Can you work these out from the drawing? Everything is in mm from the part's minimum corner. Coordinates: 2 decimals unless noted, no trailing zeros. Order: outer loops, then holes, each group sorted by start corner. A loop starts at its lowest first (then second) coordinate and runs counter-clockwise, first axis right, second up. Notation, with made-up numbers: M 39.5,65 L 80.5,65 A22 ccw 80.5,97 Z; hole C 85,65 d9. An arc over 180 degrees is marked long. Answer as CSV lines item,"result". Start each with the question number.
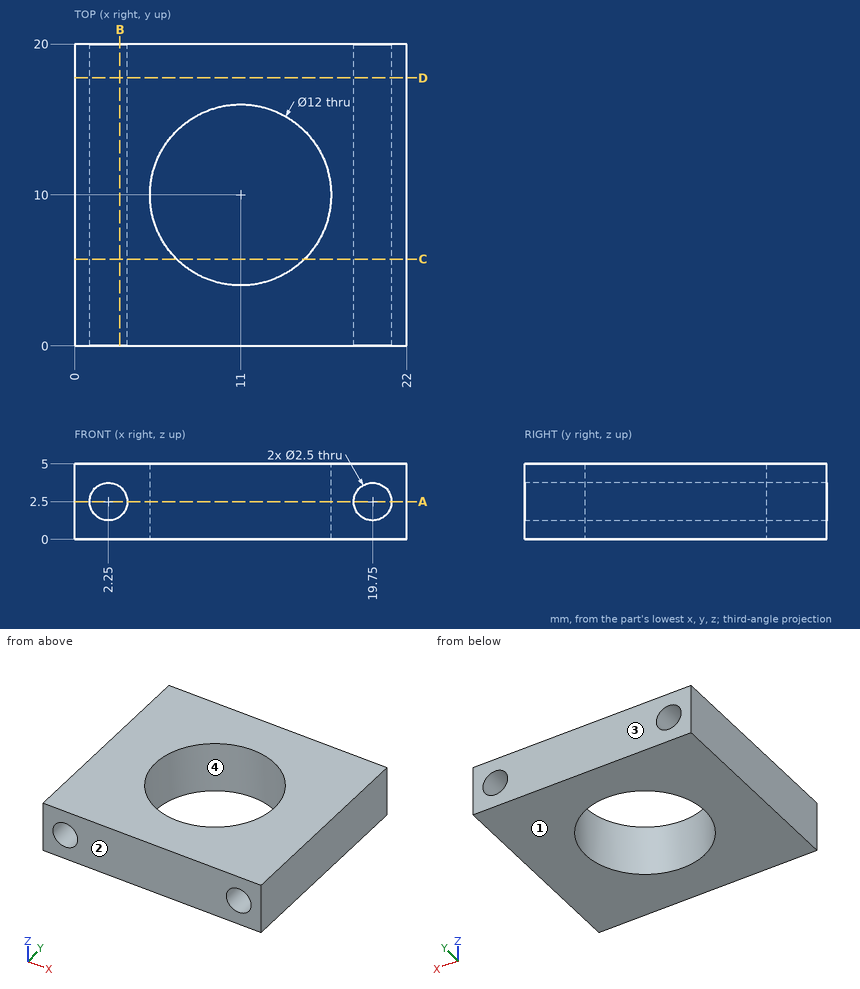
1) Will this pin go through, and if not, where does the flat tip stop? pin 1 Ø2 at (x, z) = (2.25, 2.5) entering from +Y.
2) I need wall thicknesses on line 1 (Z direction, x = 19.75, y = 14.25); line 2 (Y direction, x = 11, z = 1.9); line 3 (Y direction, x = 9.75, z = 2.7). Which ranges of each line are inside material? Lowest first, please. Write a range as [from, to].
3) Suppose I cut it at C-C on y = 5.75. Please give me the cut outline in (x, z).
4) Suppose I cut it at B-B on x = 3. Please give me the cut outline in (y, z), plus the area to 3 significant figures.
5) Suppose I cut it at D-D on y = 17.75. Please give me the cut outline in (x, z).
6) If we mould it in two halves opening along Y, with no side actions, what happens to the marked faces 1, 2, 3 and 4? For each: released by +Y, released by -Y, zero draft, split by the parting line, or undercut.
7) Suppose I cut it at A-A on z = 2.5. Please give me the cut outline in (x, y), plus the area to 3 significant figures.
Output:
1,pin 1,"through"
2,line 1,"[0, 1.25], [3.75, 5]"
2,line 2,"[0, 4], [16, 20]"
2,line 3,"[0, 4.13], [15.87, 20]"
3,outline,"M 0,0 L 6.76,0 L 6.76,5 L 0,5 Z; M 15.24,0 L 22,0 L 22,5 L 15.24,5 Z; hole C 2.25,2.5 d2.5; hole C 19.75,2.5 d2.5"
4,outline,"M 0,0 L 20,0 L 20,1.5 L 0,1.5 Z; M 0,3.5 L 20,3.5 L 20,5 L 0,5 Z"
4,area,"60.0 mm²"
5,outline,"M 0,0 L 22,0 L 22,5 L 0,5 Z; hole C 2.25,2.5 d2.5; hole C 19.75,2.5 d2.5"
6,face 1,"zero draft"
6,face 2,"released by -Y"
6,face 3,"released by +Y"
6,face 4,"undercut"
7,outline,"M 0,0 L 1,0 L 1,20 L 0,20 Z; M 3.5,0 L 18.5,0 L 18.5,20 L 3.5,20 Z; M 21,0 L 22,0 L 22,20 L 21,20 Z; hole C 11,10 d12"
7,area,"227 mm²"
